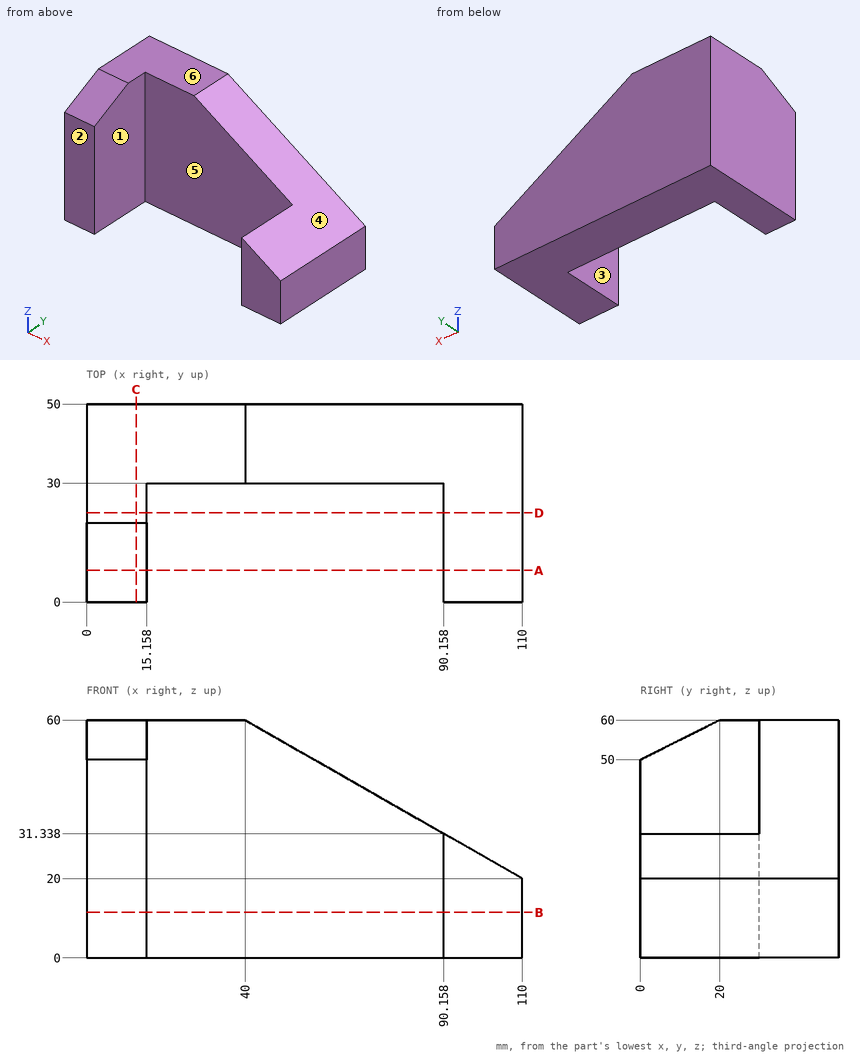
For this review, use the dimensioned drawing (mm, ordinates from the lowest corner) and the shaded views. A direction names the side the tool comes from. Round coordinates to 2 decimals unless told otherwise and drop trailing zeros. Order: outer loops, then holes, each group sorted by start corner. A loop starts at its lowest first (then second) coordinate and runs counter-clockwise, first axis right, second up. Notation, with made-up numbers: (66, 21) - (93, 21) arc R28 cw to (93, 57) - close; hole circle Ø9 at (83, 89.5). An arc over 180 degrees is marked (long way). Use one line per item in the form item = value.
Q1. Add section C-C on x = 12.5. Give the boundary of the cut face in (y, z).
Response values:
outline = (0, 0) - (50, 0) - (50, 60) - (20, 60) - (0, 50) - close
Q2. Add section B-B on z = 11.5. Give the boundary of the cut face in (x, y).
Response values:
outline = (0, 0) - (15.16, 0) - (15.16, 30) - (90.16, 30) - (90.16, 0) - (110, 0) - (110, 50) - (0, 50) - close
Q3. Tool access review of the marked faces 1 and 2: name each direction out of +Z, -Z, +X, -X, +Y, -Y from which nothing blocks a thin tool from reaching the whole face with its end or side.
Response values:
face_1 = +Z, -Z, -Y
face_2 = +Z, -Z, +X, -X, -Y
Q4. Clearance check with flat-ended pins moving along their axes: P1, Ø8, axis at x = 39, z = 39.5, coming from the -Y side; P2, Ø1, axis at y = 16, z = 44.5, coming from the +X side. State where each tip first meets the part, or that it passes through.
Response values:
P1 = 30
P2 = 15.16
Q5. Add section A-A on y = 8. Give the boundary of the cut face in (x, z), then the cut area to 3 significant figures.
Response values:
outline = (0, 0) - (15.16, 0) - (15.16, 54) - (0, 54) - close; (90.16, 0) - (110, 0) - (110, 20) - (90.16, 31.34) - close
area = 1,330 mm^2
Q6. Mouldability with a two-part tool opening along X and no side actions: class the marked faces 3, 4, 5 and 6 as pulls with the +X half, pulls with the -X half, needs draft (parallel to the pull), parting line crosses it, or undercut.
Response values:
face_3 = undercut
face_4 = pulls with the +X half
face_5 = undercut
face_6 = needs draft
Q7. Add section D-D on y = 22.5. Give the boundary of the cut face in (x, z).
Response values:
outline = (0, 0) - (15.16, 0) - (15.16, 60) - (0, 60) - close; (90.16, 0) - (110, 0) - (110, 20) - (90.16, 31.34) - close
Q8. To check wall thickness, follow line 1 (X direction, y = 9.5, z = 4); line 2 (Y direction, x = 55, z = 11); line 3 (X direction, y = 29, z = 51). State the ranges of each line that lie inside material, in increasing order.
Response values:
line_1 = 0 to 15.16, 90.16 to 110
line_2 = 30 to 50
line_3 = 0 to 15.16
